from build123d import *


with BuildPart() as f1:
    # F0 (on Front) → F1 (revolve)
    with BuildSketch(Plane.XZ):
        with BuildLine():
            Line((267.962432, 0), (0, 0))
            Line((0, 0), (0, -3.429))
            Line((0, -3.429), (266.134583, -3.429))
            ThreePointArc((266.134583, -3.429), (268.95194, -4.088218), (271.184336, -5.929))
            ThreePointArc((271.184336, -5.929), (274.622225, -8.763804), (278.960955, -9.779))
            Line((278.960955, -9.779), (292.1, -9.779))
            Line((292.1, -9.779), (292.1, -6.35))
            Line((292.1, -6.35), (278.960955, -6.35))
            ThreePointArc((278.960955, -6.35), (275.785955, -5.499261), (273.461693, -3.175))
            ThreePointArc((273.461693, -3.175), (271.137432, -0.850739), (267.962432, 0))
        make_face()
    revolve(axis=Axis((0, 0, -1.7145), (0, 0, -1)))


solid = f1.part
Work out the finished part from the listing and answer in its coordinate system (mm). A direction names the side the tool comes from. Give positions to 0.01 mm unless a question says otherwise; leave off trailing zeros. Loops run counter-clockwise (first coordinate to the right, second up) from the corner with the lowest first, then second, coordinate; pieces in that order, holes last. Notation, with made-up numbers: (35, -12) -> (87, -12) arc R16 ccw to (87, -4) -> close; hole circle Ø9 at (-28, -3.5). An arc over 180 degrees is marked (long way). Use a Markdown table: item, result. Add a question column.
1) The part is cut by section C-C, the plane z = -1.5. Determine the outline of the cut face in (x, y), plus the area to 3 significant figures.
2) Each of these flat-tipped pins is pushed along its axis until it touches: P1, Ø1, axis at x = -60.5, z = -4.5, coming from the -Y side; P2, Ø3, axis at y = 168, z = -5, coming from the -X side; P3, Ø1.5, axis at x = 144, y = -16.5, coming from the -Z side. Where does it stop, or does it pass through?
3) For a pull along X with two mould halves and no side action, classify faces 3 (the flat face through (-4, -4, 0)), 4 (the cylindrical face through (278.61, -87.74, -8.04)), 5 (the flat face through (4, -4, -3.429)) as +X half, -X half, draft (parallel to the pull), parting line (faces both ways), or undercut.
4) The part is cut by section A-A, the plane y = 0. Determine the outline of the cut face in (x, z) (3 decimals).
5) Which of the six approach directions +Z, -Z, +X, -X, +Y, -Y give full straight-line access (tool end or side, diameter ignored) to faces 1 (the flat face through (-258, 107, -9.779)), 2 (the flat face through (258, 107, -6.35))?
6) Consider line 1 along Y through (x, z) = (-7.5, -8.25); line 2 along Z through (x, y) = (191.5, -203.5); line 3 along Y through (x, z) = (-197.5, -8). Determine where each line is inside the solid, lowest interval first.
Reported:
| question | item | result |
|---|---|---|
| 1 | outline | circle Ø544.12 at (0, 0) |
| 1 | area | 233,000 mm^2 |
| 2 | P1 | stops at y = -268.32 |
| 2 | P2 | stops at x = -239.41 |
| 2 | P3 | stops at z = -3.43 |
| 3 | face 3 | draft |
| 3 | face 4 | parting line |
| 3 | face 5 | undercut |
| 4 | outline | (-292.1, -9.779) -> (-278.961, -9.779) arc R9.779 ccw to (-271.184, -5.929) arc R6.35 cw to (-266.135, -3.429) -> (266.135, -3.429) arc R6.35 cw to (271.184, -5.929) arc R9.779 ccw to (278.961, -9.779) -> (292.1, -9.779) -> (292.1, -6.35) -> (278.961, -6.35) arc R6.35 cw to (273.462, -3.175) arc R6.35 ccw to (267.962, 0) -> (-267.962, 0) arc R6.35 ccw to (-273.462, -3.175) arc R6.35 cw to (-278.961, -6.35) -> (-292.1, -6.35) -> close |
| 5 | face 1 | -Z, +X, -X, +Y, -Y |
| 5 | face 2 | +Z |
| 6 | line 1 | y = -292 to -273.61, 273.61 to 292 |
| 6 | line 2 | z = -9.78 to -6.35 |
| 6 | line 3 | y = -215.21 to -188.96, 188.96 to 215.21 |
